```python
from build123d import *

# Parameters (mm, degrees)
F0_W      = 61.3026209176
F0_H      = 111.3808304071
F1_DEPTH  = 8.89
F2_W      = 61.3026209176
F2_H      = 13.814676553
F3_DEPTH  = 18.796
F5_DEPTH  = 13.97
F6_W      = 23.2926858589
F6_H      = 41.1077216268
F7_DEPTH  = 25.4
F9_DEPTH  = 25.4
F10_W     = 6.8394243717
F10_H     = 10.9558589756
F11_DEPTH = 25.4
F12_W     = 8.89
F12_H     = 6.8394243717
F13_DEPTH = 25.4
F14_W     = 9.398
F14_H     = 6.8394243717
F15_DEPTH = 25.4


with BuildPart() as f1:
    # F0 (on Right) → F1 (new body)
    with BuildSketch(Plane.YZ):
        Rectangle(F0_W, F0_H)
    extrude(amount=F1_DEPTH)

    # F2 (on face) → F3 (join)
    with BuildSketch(Plane.YZ.offset(8.89)):
        with Locations((0, -48.7830769271)):
            Rectangle(F2_W, F2_H)
    extrude(amount=F3_DEPTH)

    # F4 (on face) → F5 (join)
    with BuildSketch(Plane.XY.offset(-41.8757386506)):
        with BuildLine():
            Line((27.686, 30.6513104588), (27.686, -30.6513104588))
            ThreePointArc((27.686, -30.6513104588), (47.0533316353, 0), (27.686, 30.6513104588))
        make_face()
    extrude(amount=-F5_DEPTH)

    # F6 (on face) → F7 (cut)
    with BuildSketch(Plane.YZ.offset(8.89)):
        with Locations((0.7317778654, 35.1365543902)):
            Rectangle(F6_W, F6_H)
    extrude(amount=-F7_DEPTH, mode=Mode.SUBTRACT)

    # F8 (on face) → F9 (cut)
    with BuildSketch(Plane.YZ.offset(8.89)):
        with BuildLine():
            Line((12.3781207949, 14.5826935768), (-10.914565064, 14.5826935768))
            ThreePointArc((-10.914565064, 14.5826935768), (0.7317778654, 2.9363506474), (12.3781207949, 14.5826935768))
        make_face()
    extrude(amount=-F9_DEPTH, mode=Mode.SUBTRACT)

    # F10 (on face) → F11 (cut)
    with BuildSketch(Plane.YZ.offset(8.89)):
        with Locations((27.2315982729, -36.3978091627)):
            Rectangle(F10_W, F10_H)
    extrude(amount=-F11_DEPTH, mode=Mode.SUBTRACT)

    # F12 (on face) → F13 (cut)
    with BuildSketch(Plane.XY.offset(-41.8757386506)):
        with Locations((4.445, 27.2315982729)):
            Rectangle(F12_W, F12_H)
    extrude(amount=-F13_DEPTH, mode=Mode.SUBTRACT)

    # F14 (on face) → F15 (cut)
    with BuildSketch(Plane.XY.offset(-41.8757386506)):
        with Locations((13.589, 27.2315982729)):
            Rectangle(F14_W, F14_H)
    extrude(amount=-F15_DEPTH, mode=Mode.SUBTRACT)


solid = f1.part
```
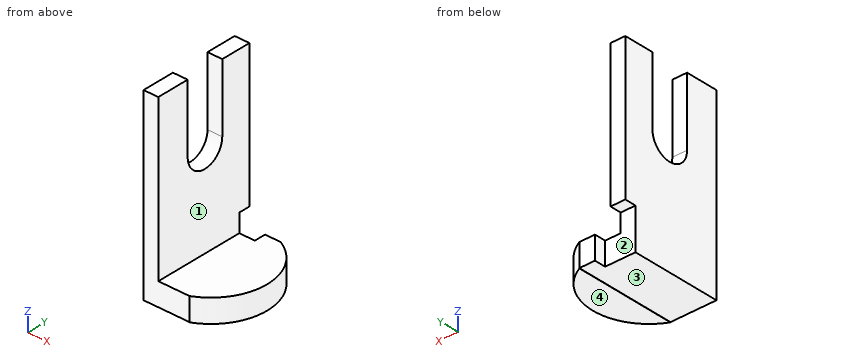
Verification items for the finished model (mm, model axes). Face numbers are marked on the shaded views. A direction names the side the tool comes from. Round coordinates to 2 decimals unless told otherwise and drop trailing zeros. Order: outer loops, then holes, each group sorted by start corner. A loop starts at its lowest first (then second) coordinate and runs counter-clockwise, first axis right, second up. Notation, with made-up numbers: (-32.5, 1) - (-7.5, 1) arc R18 ccw to (-7.5, 34) - close; hole circle Ø5 at (76.5, -33.75). An arc over 180 degrees is marked (long way). Use CSV: the item, a comma, the result in double quotes. Start each with the question number.
1) Section check D-D, the plane z = -40. Record the cut outline in (x, y), plus the area to 3 significant figures.
2) Section check B-B, the plane x = 6.5. Record the cut outline in (y, z).
3) Access from +Z, -Z, +X, -X, +Y, -Y to the whole of each face (thin tool, end or side, straight path). Record for the marked faces 1, 2, 3 and 4.
4) Section check C-C, the plane y = 1.5. Record the cut outline in (x, z).
5) Section check A-A, the plane z = 25. Record the cut outline in (x, y).
6) Go/stop test with flat-tipped pins: P1, Ø14, axis at x = 9.5, y = -14, coming from the -Z side; P2, Ø4, axis at y = -10, z = 25, coming from the -X side; P3, Ø5.5, axis at x = 10.5, z = -47, coming from the +Y side; P4, Ø12, axis at y = 18.5, z = -33, coming from the +X side. Record where each tip stops, or that it passes through.
7) Thickness scan on L1, parallel to Y at x = 3.5, z = 34; L2, parallel to X at y = -5, z = -21; L3, parallel to Z at x = 15, y = 0. Record the ranges inside material, lowest first.
Answers:
1,outline,"(0, -30.65) - (8.89, -30.65) - (8.89, 23.81) - (0, 23.81) - close"
1,area,"484 mm²"
2,outline,"(-30.65, -55.69) - (23.81, -55.69) - (23.81, -30.92) - (30.65, -30.92) - (30.65, 55.69) - (12.38, 55.69) - (12.38, 14.58) arc R11.65 cw to (-10.91, 14.58) - (-10.91, 55.69) - (-30.65, 55.69) - close"
3,face 1,"+Z, +X, +Y, -Y"
3,face 2,"-Z, -X, +Y"
3,face 3,"-Z, -X, +Y, -Y"
3,face 4,"-Z, +X, -X, +Y, -Y"
4,outline,"(0, -55.69) - (27.69, -55.69) - (27.69, -55.85) - (47.02, -55.85) - (47.02, -41.88) - (8.89, -41.88) - (8.89, 2.96) - (0, 2.96) - close"
5,outline,"(0, -30.65) - (8.89, -30.65) - (8.89, -10.91) - (0, -10.91) - close; (0, 12.38) - (8.89, 12.38) - (8.89, 30.65) - (0, 30.65) - close"
6,P1,"stops at z = -55.69"
6,P2,"stops at x = 0"
6,P3,"stops at y = 23.81"
6,P4,"stops at x = 8.89"
7,L1,"y = -30.65 to -10.91, 12.38 to 30.65"
7,L2,"x = 0 to 8.89"
7,L3,"z = -55.69 to -41.88"
